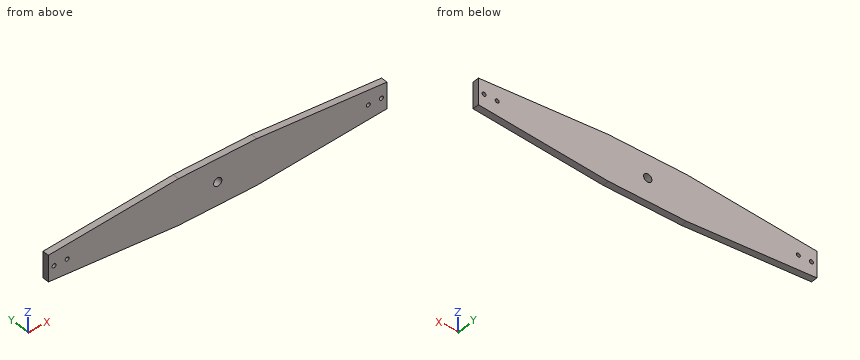
from build123d import *

# Parameters (mm, degrees)
SKETCH1_R           = 3
SKETCH1_R_2         = 6.35
BOSS_EXTRUDE1_DEPTH = 10


with BuildPart() as part:
    # Sketch1 → Boss-Extrude1 (new body)
    with BuildSketch(Plane(origin=(0, 0, 0), x_dir=(1, 0, 0), z_dir=(0, 1, 0))):
        Polygon((-60, 34.925), (60, 34.925), (259.43812075, 19.943812075), (259.43812075, -19.943812075), (60, -34.925), (-60, -34.925), (-259.43812075, -19.943812075), (-259.43812075, 19.943812075), align=None)
        with Locations((-250.825, 0)):
            Circle(SKETCH1_R, mode=Mode.SUBTRACT)
        with Locations((250.825, 0)):
            Circle(SKETCH1_R, mode=Mode.SUBTRACT)
        Circle(SKETCH1_R_2, mode=Mode.SUBTRACT)
        with Locations((-230.825, 0)):
            Circle(SKETCH1_R, mode=Mode.SUBTRACT)
        with Locations((230.825, 0)):
            Circle(SKETCH1_R, mode=Mode.SUBTRACT)
    extrude(amount=BOSS_EXTRUDE1_DEPTH)


solid = part.part
The model under review builds one solid part; all positions refer to its coordinate system, in mm. Round coordinates to 2 decimals unless told otherwise and drop trailing zeros. Loops run counter-clockwise (first coordinate to the right, second up) from the corner with the lowest first, then second, coordinate; pieces in that order, holes last. Notation, with made-up numbers: (-11.5, 77.25) -> (18.5, 77.25) arc R27 cw to (18.5, 99.25) -> close; hole circle Ø9 at (45, 55). An arc over 180 degrees is marked (long way). Write item = value, one per line. Start each with the question number.
Item 1: Take a section at D-D on z = -25.5. Give the boundary of the cut face in (x, y), plus the area to 3 significant figures.
Item 2: Take a section at B-B on y = 2.75. Give the boundary of the cut face in (x, z) (3 decimals), plus the area to 3 significant figures.
Item 3: Take a section at C-C on x = 147. Give the boundary of the cut face in (y, z), plus the area to 3 significant figures.
Item 4: Insertion check: pin 1 (1 mm diameter, centred on x = 100.5, y = 5, fed in from -Z); pin 2 (5 mm diameter, centred on x = -157.5, y = 8.5, fed in from +Z). Each pin has a flat end and moves straight along its axis. Give the tip position at first contact, or say it passes through.
Item 5: To check wall thickness, follow L1, parallel to X at y = 5, z = 0 (3 decimals); L2, parallel to Z at x = 0, y = 5.25 (3 decimals); L3, parallel to Z at x = -5, y = 2 (3 decimals). State the ranges of each line that lie inside material, in increasing order.
Item 6: Take a section at A-A on x = 0. Give the boundary of the cut face in (y, z) (3 decimals), plus the area to 4 significant figures.
Result:
q1.outline = (-185.47, 0) -> (185.47, 0) -> (185.47, 10) -> (-185.47, 10) -> close
q1.area = 3,710 mm²
q2.outline = (-259.438, -19.944) -> (-60, -34.925) -> (60, -34.925) -> (259.438, -19.944) -> (259.438, 19.944) -> (60, 34.925) -> (-60, 34.925) -> (-259.438, 19.944) -> close; hole circle Ø6 at (-250.825, 0); hole circle Ø6 at (-230.825, 0); hole circle Ø12.7 at (0, 0); hole circle Ø6 at (230.825, 0); hole circle Ø6 at (250.825, 0)
q2.area = 30,000 mm²
q3.outline = (0, -28.39) -> (10, -28.39) -> (10, 28.39) -> (0, 28.39) -> close
q3.area = 568 mm²
q4.pin_1 = -31.92
q4.pin_2 = 27.79
q5.L1 = -259.438 to -253.825, -247.825 to -233.825, -227.825 to -6.35, 6.35 to 227.825, 233.825 to 247.825, 253.825 to 259.438
q5.L2 = -34.925 to -6.35, 6.35 to 34.925
q5.L3 = -34.925 to -3.914, 3.914 to 34.925
q6.outline = (0, -34.925) -> (10, -34.925) -> (10, -6.35) -> (0, -6.35) -> close; (0, 6.35) -> (10, 6.35) -> (10, 34.925) -> (0, 34.925) -> close
q6.area = 571.5 mm²
